```python
from build123d import *

# Parameters (mm, degrees)
SKETCH_1_R      = 10
SKETCH_1_R_2    = 1.5
EXTRUDE_1_DEPTH = 2
SKETCH_2_R      = 4.5
SKETCH_2_R_2    = 2.75
EXTRUDE_2_DEPTH = 2.5


with BuildPart() as part:
    # 草图1 → 凸台-拉伸1 (new body)
    with BuildSketch(Plane(origin=(0, 0, 0), x_dir=(1, 0, 0), z_dir=(0, 1, 0))):
        with Locations(Location((0, 0, 0), (0, 0, 270))):
            Circle(SKETCH_1_R)
        with Locations(Location((-7, 0, 0), (0, 0, 270))):
            Circle(SKETCH_1_R_2, mode=Mode.SUBTRACT)
        with Locations(Location((0, 7, 0), (0, 0, 270))):
            Circle(SKETCH_1_R_2, mode=Mode.SUBTRACT)
        with Locations(Location((7, 0, 0), (0, 0, 270))):
            Circle(SKETCH_1_R_2, mode=Mode.SUBTRACT)
        with Locations(Location((0, -7, 0), (0, 0, 270))):
            Circle(SKETCH_1_R_2, mode=Mode.SUBTRACT)
        with Locations(Location((0, 0, 0), (0, 0, 270))):
            Circle(SKETCH_1_R_2, mode=Mode.SUBTRACT)
    extrude(amount=EXTRUDE_1_DEPTH)

    # 草图2 → 凸台-拉伸2 (add)
    with BuildSketch(Plane(origin=(0, 0, 0), x_dir=(1, 0, 0), z_dir=(0, 1, 0))):
        with Locations(Location((0, 0, 0), (0, 0, 270))):
            Circle(SKETCH_2_R)
        with Locations(Location((0, 0, 0), (0, 0, 270))):
            Circle(SKETCH_2_R_2, mode=Mode.SUBTRACT)
    extrude(amount=-EXTRUDE_2_DEPTH)


solid = part.part
```
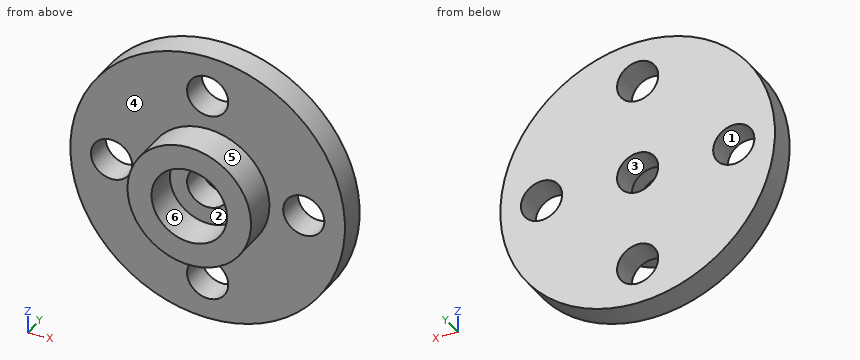
Geometry check sheet. Reference: the model listing, model coordinates, mm. Face numbers are marked on the shaded views. A direction names the side the tool comes from. Round coordinates to 2 decimals unless told otherwise and drop trailing zeros. Order: outer loops, then holes, each group sorted by start corner. A loop starts at its lowest first (then second) coordinate and runs counter-clockwise, first axis right, second up. Notation, with made-up numbers: (84, 82.25) - (128, 82.25) arc R22 ccw to (128, 90.25) - close; hole circle Ø9 at (-28, -6.5). An arc over 180 degrees is marked (long way). Use a Markdown table: item, result. Add a question column.
(1) Sectioned sample at C-C, the plane z = -7.5. Enter the section's corners in (x, y).
(2) Depth check by flat-ended pin: pin 1 (2 mm diameter, centred on y = 1, z = -8, fed in from -X); pin 2 (3 mm diameter, centred on x = -8, z = 1, fed in from -Y). Enter the tip coordinate at first touch or a pass-through.
(3) Material ranges on line 1 along X through (y, z) = (1.1, 0); line 2 along Z through (x, y) = (-1.25, 1.6); line 3 along X through (y, z) = (-1.2, 0), recorded low to high. Write a range as [from, to].
(4) Sectioned sample at B-B, the plane z = 0. Enter the section's corners in (x, y).
(5) Tool access check on the marked faces 1 and 2. Record the directions out of +Z, -Z, +X, -X, +Y, -Y that give a thin tool (end or side, any length) a straight path to the whole face; none if there is none.
(6) Sectioned sample at A-A, the plane x = 0. Enter the section's corners in (y, z), and give its area (4 significant figures).
(7) Release check for a two-part mould opening along X. For the marked faces 3, 4, 5 and 6 record: pulls with the +X half, pulls with the -X half, needs draft (parallel to the pull), parting line crosses it, or undercut.
(8) Sectioned sample at D-D, the plane y = 0.9. Enter the section's corners in (x, z).
Answers below:
| question | item | result |
|---|---|---|
| 1 | outline | (-6.61, 0) - (-1.41, 0) - (-1.41, 2) - (-6.61, 2) - close; (1.41, 0) - (6.61, 0) - (6.61, 2) - (1.41, 2) - close |
| 2 | pin 1 | x = -7.14 |
| 2 | pin 2 | y = 0 |
| 3 | line 1 | [-10, -8.5], [-5.5, -1.5], [1.5, 5.5], [8.5, 10] |
| 3 | line 2 | [-9.92, -7.83], [-6.17, -0.83], [0.83, 6.17], [7.83, 9.92] |
| 3 | line 3 | [-4.5, -2.75], [2.75, 4.5] |
| 4 | outline | (-10, 0) - (-8.5, 0) - (-8.5, 2) - (-10, 2) - close; (-5.5, 0) - (-4.5, 0) - (-4.5, -2.5) - (-2.75, -2.5) - (-2.75, 0) - (-1.5, 0) - (-1.5, 2) - (-5.5, 2) - close; (1.5, 0) - (2.75, 0) - (2.75, -2.5) - (4.5, -2.5) - (4.5, 0) - (5.5, 0) - (5.5, 2) - (1.5, 2) - close; (8.5, 0) - (10, 0) - (10, 2) - (8.5, 2) - close |
| 5 | face 1 | +Y, -Y |
| 5 | face 2 | -Y |
| 6 | outline | (-2.5, -4.5) - (0, -4.5) - (0, -5.5) - (2, -5.5) - (2, -1.5) - (0, -1.5) - (0, -2.75) - (-2.5, -2.75) - close; (-2.5, 2.75) - (0, 2.75) - (0, 1.5) - (2, 1.5) - (2, 5.5) - (0, 5.5) - (0, 4.5) - (-2.5, 4.5) - close; (0, -10) - (2, -10) - (2, -8.5) - (0, -8.5) - close; (0, 8.5) - (2, 8.5) - (2, 10) - (0, 10) - close |
| 6 | area | 30.75 mm² |
| 7 | face 3 | undercut |
| 7 | face 4 | needs draft |
| 7 | face 5 | parting line crosses it |
| 7 | face 6 | undercut |
| 8 | outline | circle Ø20 at (0, 0); hole circle Ø3 at (-7, 0); hole circle Ø3 at (0, -7); hole circle Ø3 at (0, 0); hole circle Ø3 at (0, 7); hole circle Ø3 at (7, 0) |
